Geometry check sheet. Reference: the model listing, model coordinates, mm. Give positions to 0.01 mm unless a question says otherwise; leave off trailing zeros. Loops run counter-clockwise (first coordinate to the right, second up) from the corner with the lowest first, then second, coordinate; pieces in that order, holes last. Notation, with made-up numbers: (9, 37.5) -> (41, 37.5) arc R13 cw to (41, 42.5) -> close; hole circle Ø1 at (69.5, 83.5). An arc over 180 degrees is marked (long way). One line per item, written item: value. Start each with the question number.
(1) Gauge pin test, flat ends, axial feed: pin 1 Ø1.5 at (y, z) = (-2.5, 23.5) entering from +X; pin 2 Ø3 at (x, z) = (2.5, 6) entering from -Y. Record the tip position at first contact, or that the pin passes through.
(2) Sectioned sample at A-A, the plane x = 0. Record the cut outline in (y, z), then the cut area to 4 significant figures.
(3) Sectioned sample at D-D, the plane z = 22. Record the cut outline in (x, y).
(4) Scan lines: line 1 along Z through (x, y) = (0, 1.25); line 2 along X through (y, z) = (0.25, 7.5); line 3 along X through (y, z) = (-0.75, 22). Record each from-to range of solid material in increasing order. Write a range as from..to.
(5) Sectioned sample at B-B, the plane y = 0. Record the cut outline in (x, z).
(6) Sectioned sample at C-C, the plane z = 7. Record the cut outline in (x, y), then the cut area to 3 significant figures.
from build123d import *

# Parameters (mm, degrees)
SKETCH1_R               = 8
BOSS_EXTRUDE1_DEPTH     = 44
SKETCH2_R               = 2.5
CUT_EXTRUDE1_DEPTH      = 9
CUT_EXTRUDE1_DEPTH_BACK = 9
CHAMFER1_SIZE           = 0.5


with BuildPart() as part:
    # Sketch1 → Boss-Extrude1 (new body)
    with BuildSketch(Plane.XY):
        Circle(SKETCH1_R)
    extrude(amount=BOSS_EXTRUDE1_DEPTH)

    # Sketch2 → Cut-Extrude1 (cut, two sides)
    with BuildSketch(Plane(origin=(0, 0, 0), x_dir=(1, 0, 0), z_dir=(0, 1, 0))) as cut_extrude1_sk:
        with Locations((0, -22)):
            Circle(SKETCH2_R)
    extrude(amount=CUT_EXTRUDE1_DEPTH, mode=Mode.SUBTRACT)
    extrude(cut_extrude1_sk.sketch, amount=-CUT_EXTRUDE1_DEPTH_BACK, mode=Mode.SUBTRACT)

    # Chamfer1
    chamfer1_edges = [part.edges().sort_by_distance(p)[0] for p in [
        (-8, 0, 0),
        (-8, 0, 44),
    ]]
    chamfer(chamfer1_edges, length=CHAMFER1_SIZE)


solid = part.part
Calculated:
1. pin 1: stops at x = 7.81
1. pin 2: stops at y = -7.94
2. outline: (-8, 0.5) -> (-7.5, 0) -> (7.5, 0) -> (8, 0.5) -> (8, 19.5) -> (-8, 19.5) -> close; (-8, 24.5) -> (8, 24.5) -> (8, 43.5) -> (7.5, 44) -> (-7.5, 44) -> (-8, 43.5) -> close
2. area: 623.5 mm2
3. outline: (-2.5, -7.6) -> (-2.5, 7.6) arc R8 ccw to start; (2.5, -7.6) arc R8 ccw to (2.5, 7.6) -> close
4. line 1: z = 0..19.5, 24.5..44
4. line 2: x = -8..8
4. line 3: x = -7.96..-2.5, 2.5..7.96
5. outline: (-8, 0.5) -> (-7.5, 0) -> (7.5, 0) -> (8, 0.5) -> (8, 43.5) -> (7.5, 44) -> (-7.5, 44) -> (-8, 43.5) -> close; hole circle Ø5 at (0, 22)
6. outline: circle Ø16 at (0, 0)
6. area: 201 mm2
